Geometry: final body of the model. Coordinates: model frame, mm. Round coordinates to 2 decimals unless told otherwise and drop trailing zeros. Loops run counter-clockwise (first coordinate to the right, second up) from the corner with the lowest first, then second, coordinate; pieces in that order, holes last. Notation, with made-up numbers: (-29, 77) - (-13, 77) arc R19 ccw to (-13, 84) - close; hole circle Ø6 at (87, -40). An arc over 180 degrees is marked (long way). Use CSV: the item, a comma, the result in double quotes.
Autodesk Inventor part; units mm, degrees
ref_plane "Work Plane3" through (0, -20, 0) normal (0, 1, 0) x (-1, 0, 0)
ref_plane "YZ Plane" through (0, 0, 0) normal (1, 0, 0) x (0, 1, 0)
ref_plane "XY Plane" through (0, 0, 0) normal (0, 0, 1) x (1, 0, 0)
sketch "Sketch1" plane through (0, 0, 0) normal (0, 0, 1) x (1, 0, 0)
  line L0 (-3.9007, 3.9007) -> (3.9007, 3.9007)
  line L1 (3.9007, 3.9007) -> (3.9007, -3.9007)
  line L2 (3.9007, -3.9007) -> (-3.9007, -3.9007)
  line L3 (-3.9007, -3.9007) -> (-3.9007, 3.9007)
  line L4 (0, 3.9007) -> (0, -3.9007) construction
  line L5 (-3.9007, 0) -> (3.9007, 0) construction
  circle A0 centre (0, 0) radius 2.1
  line L6 (0, 0) -> (-16.1173, 16.1173) construction
  line L7 (0, 0) -> (22.7933, 0) construction
  line L8 (-2.84, 3.9007) -> (-5.4993, 6.56)
  line L9 (-5.4993, 6.56) -> (-5.4993, 8.2)
  line L10 (-5.4993, 8.2) -> (-2.84, 8.2)
  line L11 (-2.84, 8.2) -> (-4.64, 10)
  line L12 (-4.64, 10) -> (-10, 10)
  line L13 (-10, 10) -> (-10, 4.64)
  line L14 (-10, 4.64) -> (-8.2, 2.84)
  line L15 (-8.2, 2.84) -> (-8.2, 5.4993)
  line L16 (-8.2, 5.4993) -> (-6.56, 5.4993)
  line L17 (-6.56, 5.4993) -> (-3.9007, 2.84)
  line L18 (-3.9007, 2.84) -> (-11.3102, 2.84) construction
  line L19 (-2.84, 3.9007) -> (-3.9007, 3.9007)
  line L20 (-3.9007, 2.84) -> (-3.9007, 3.9007)
  line L21 (-3.9007, -2.84) -> (-6.56, -5.4993)
  line L22 (-6.56, -5.4993) -> (-8.2, -5.4993)
  line L23 (-8.2, -5.4993) -> (-8.2, -2.84)
  line L24 (-8.2, -2.84) -> (-10, -4.64)
  line L25 (-10, -4.64) -> (-10, -10)
  line L26 (-10, -10) -> (-4.64, -10)
  line L27 (-4.64, -10) -> (-2.84, -8.2)
  line L28 (-2.84, -8.2) -> (-5.4993, -8.2)
  line L29 (-5.4993, -8.2) -> (-5.4993, -6.56)
  line L30 (-5.4993, -6.56) -> (-2.84, -3.9007)
  line L31 (-3.9007, -2.84) -> (-3.9007, -3.9007)
  line L32 (-2.84, -3.9007) -> (-3.9007, -3.9007)
  line L33 (2.84, -3.9007) -> (5.4993, -6.56)
  line L34 (5.4993, -6.56) -> (5.4993, -8.2)
  line L35 (5.4993, -8.2) -> (2.84, -8.2)
  line L36 (2.84, -8.2) -> (4.64, -10)
  line L37 (4.64, -10) -> (10, -10)
  line L38 (10, -10) -> (10, -4.64)
  line L39 (10, -4.64) -> (8.2, -2.84)
  line L40 (8.2, -2.84) -> (8.2, -5.4993)
  line L41 (8.2, -5.4993) -> (6.56, -5.4993)
  line L42 (6.56, -5.4993) -> (3.9007, -2.84)
  line L43 (2.84, -3.9007) -> (3.9007, -3.9007)
  line L44 (3.9007, -2.84) -> (3.9007, -3.9007)
  line L45 (3.9007, 2.84) -> (6.56, 5.4993)
  line L46 (6.56, 5.4993) -> (8.2, 5.4993)
  line L47 (8.2, 5.4993) -> (8.2, 2.84)
  line L48 (8.2, 2.84) -> (10, 4.64)
  line L49 (10, 4.64) -> (10, 10)
  line L50 (10, 10) -> (4.64, 10)
  line L51 (4.64, 10) -> (2.84, 8.2)
  line L52 (2.84, 8.2) -> (5.4993, 8.2)
  line L53 (5.4993, 8.2) -> (5.4993, 6.56)
  line L54 (5.4993, 6.56) -> (2.84, 3.9007)
  line L55 (3.9007, 2.84) -> (3.9007, 3.9007)
  line L56 (2.84, 3.9007) -> (3.9007, 3.9007)
  dimension "d7" = 4.2
  dimension "d8" = 135
  dimension "d9" = 1.5
  dimension "d10" = 1.64
  dimension "d11" = 1.8
  dimension "d12" = 2.84
  dimension "d13" = 10
  dimension "d16" = 360
extrude "Extrusion1" add sketch "Sketch1" along normal blind 160
pattern_linear "Rectangular Pattern1" count 2 spacing 20 along (0, -1, 0) of "Extrusion1"
sketch "Sketch2" plane through (0, 0, 160) normal (0, 0, 1) x (1, 0, 0)
  line L0 (8.2, -2.84) -> (8.2, -5.4993)
  line L1 (8.2, -5.4993) -> (6.56, -5.4993)
  line L2 (-6.56, -5.4993) -> (-8.2, -5.4993)
  line L3 (-8.2, -5.4993) -> (-8.2, -2.84)
  line L4 (-8.2, -14.5007) -> (-6.56, -14.5007)
  line L5 (6.56, -14.5007) -> (8.2, -14.5007)
  line L6 (5.4993, -11.8) -> (5.4993, -13.44)
  line L7 (5.4993, -13.44) -> (2.84, -16.0993)
  line L8 (-2.84, -16.0993) -> (-5.4993, -13.44)
  line L9 (-5.4993, -8.2) -> (-5.4993, -6.56)
  line L10 (-5.4993, -6.56) -> (-2.84, -3.9007)
  line L11 (2.84, -3.9007) -> (5.4993, -6.56)
  line L12 (2.84, -8.2) -> (4.64, -10)
  line L13 (-8.2, -6.9993) -> (-5.9387, -6.9993)
  line L14 (-5.9387, -6.9993) -> (-4.1231, -5.1837)
  line L15 (-4.1231, -5.1837) -> (4.1231, -5.1837)
  line L16 (4.1231, -5.1837) -> (5.9387, -6.9993)
  line L17 (5.9387, -6.9993) -> (8.2, -6.9993)
  line L18 (8.2, -6.9993) -> (8.2, -13.0007)
  line L19 (8.2, -13.0007) -> (5.9387, -13.0007)
  line L20 (5.9387, -13.0007) -> (4.2461, -14.6932)
  line L21 (4.2461, -14.6932) -> (-4.2461, -14.6932)
  line L22 (-4.2461, -14.6932) -> (-5.9387, -13.0007)
  line L23 (-5.9387, -13.0007) -> (-8.2, -13.0007)
  line L24 (-8.2, -13.0007) -> (-8.2, -6.9993)
  dimension "d23" = 1.5
  dimension "d24" = 1.5
  dimension "d25" = 1.5
  dimension "d26" = 1.5
extrude "Extrusion2" cut sketch "Sketch2" against normal up to next
ref_plane "Work Plane3" through (0, -20, 0) normal (0, 1, 0) x (-1, 0, 0)
ref_plane "Work Plane2" through (0, 0, 0) normal (0, 1, 0) x (-1, 0, 0)
ref_plane "Work Plane1" through (0, -10, 0) normal (0, 1, 0) x (-1, 0, 0)
equation "\"d24\" = d23"
equation "\"d25\" = d23"
equation "\"d26\" = d23"
properties part number "20x40x597mm" material "Aluminum 6061"
Item 1: Section C-C on z = 50. Give the number of separate pieces and of enclosed holes in the cut face, plus the area to 3 significant figures.
Final values:
separate pieces,"1"
enclosed holes,"3"
area,"297 mm²"
Item 2: Section B-B on x = 0. Return the cut outline in (y, z).
Final values:
outline,"(-23.9, 0) - (-22.1, 0) - (-22.1, 160) - (-23.9, 160) - close; (-17.9, 0) - (-16.1, 0) - (-16.1, 160) - (-17.9, 160) - close; (-3.9, 0) - (-2.1, 0) - (-2.1, 160) - (-3.9, 160) - close; (2.1, 0) - (3.9, 0) - (3.9, 160) - (2.1, 160) - close"
Item 3: Pin query (flat end, axial travel): P1, Ø3, axis at y = 1.5, z = 51, coming from the +X side; P2, Ø1.5, axis at y = -0.5, z = 45.5, coming from the +X side; P3, Ø2, axis at y = -16.5, z = 60.5, coming from the -X side; P4, Ø6, axis at x = 1, y = -7, coming from the -Z side. Return the tip coordinate at first contact, or that it passes through.
Final values:
P1,"stops at x = 8.36"
P2,"stops at x = 3.9"
P3,"stops at x = -9.86"
P4,"passes through"
Item 4: Material intervals for line 1 (Y direction, x = 0, z = 108); line 2 (X direction, y = 7, z = 149); line 3 (Y direction, x = 7.5, z = 140), sorted ascending.
Final values:
line 1,"y = -23.9 to -22.1, -17.9 to -16.1, -3.9 to -2.1, 2.1 to 3.9"
line 2,"x = -10 to -5.5, 5.5 to 10"
line 3,"y = -30 to -25.5, -14.5 to -13, -7 to -5.5, 5.5 to 10"
Item 5: Mould query, pull axis X, two halves, no side actions, for faces 1 (the flat face through (0, -23.901, 79)), 2 (the flat face through (-5, -5, 0)), 3 (the flat face through (3.901, 0, 79)), 4 (the flat face through (8.2, -24, 79)). Classes: released by +X, released by -X, zero draft, split by the parting line, or undercut.
Final values:
face 1,"undercut"
face 2,"zero draft"
face 3,"released by +X"
face 4,"undercut"
Item 6: Section A-A on y = -20. Return the cut outline in (x, z), plus the area to 3 significant figures.
Final values:
outline,"(-3.9, 0) - (-2.1, 0) - (-2.1, 160) - (-3.9, 160) - close; (2.1, 0) - (3.9, 0) - (3.9, 160) - (2.1, 160) - close"
area,"576 mm²"
